from build123d import *

# Parameters (mm, degrees)
SKETCH1_W               = 36
SKETCH1_H               = 36
BOSS_EXTRUDE1_DEPTH     = 6.5
SKETCH2_R               = 14
SKETCH2_R_2             = 5.9
BOSS_EXTRUDE2_DEPTH     = 9.15
CAVITY1_START           = 5.65
CAVITY1_OUTLINE_R       = 5.4
CAVITY1_DEPTH           = 10
SKETCH5_W               = 36
SKETCH5_H               = 36
CUT_EXTRUDE1_DEPTH      = 8.55
SKETCH6_R               = 1.83
CUT_EXTRUDE2_DEPTH      = 2.1
FILLET1_R               = 1
CUT_EXTRUDE3_DEPTH      = 28.349588662
CUT_EXTRUDE3_DEPTH_BACK = 28.349588662
SKETCH7_R               = 0.665


with BuildPart() as part:
    # Sketch1 → Boss-Extrude1 (new, symmetric)
    with BuildSketch(Plane(origin=(0, 0, 0), x_dir=(1, 0, 0), z_dir=(0, 1, 0))):
        Rectangle(SKETCH1_W, SKETCH1_H)
    extrude(amount=BOSS_EXTRUDE1_DEPTH, both=True)

    # Sketch2 → Boss-Extrude2 (add)
    with BuildSketch(Plane(origin=(0, 6.5, 0), x_dir=(1, 0, 0), z_dir=(0, 1, 0))):
        with Locations(Location((0, 0, 0), (0, 0, 270))):
            Circle(SKETCH2_R)
        with Locations(Location((0, 0, 0), (0, 0, 270))):
            Circle(SKETCH2_R_2, mode=Mode.SUBTRACT)
    extrude(amount=BOSS_EXTRUDE2_DEPTH)

    # Cavity1: read off the stored shape, not the designer's step
    # Cavity1 outline → Cavity1 (cut)
    with BuildSketch(Plane(origin=(0, 0, 0), x_dir=(1, 0, 0), z_dir=(0, 1, 0)).offset(CAVITY1_START)):
        with BuildLine():
            Line((-4.533292403, -11.068981767), (-1.149066665, -7.035818585))
            ThreePointArc((-1.149066665, -7.035818585), (0.633927393, -6.640538319), (1.47721163, -8.260472267))
            Line((1.47721163, -8.260472267), (0.68813613, -12.7355418))
            ThreePointArc((0.68813613, -12.7355418), (0.138338934, -13.654010782), (-0.883764559, -13.972077877))
            ThreePointArc((-0.883764559, -13.972077877), (1.633368507, -13.904391656), (4.097662599, -13.3869026))
            ThreePointArc((4.097662599, -13.3869026), (2.691904846, -13.099521272), (2.170695102, -11.762702927))
            Line((2.170695102, -11.762702927), (2.83719432, -6.540139582))
            ThreePointArc((2.83719432, -6.540139582), (4.123439724, -5.243649297), (5.708657981, -6.150510574))
            Line((5.708657981, -6.150510574), (7.46425068, -10.341785051))
            ThreePointArc((7.46425068, -10.341785051), (7.498293668, -11.411693133), (6.810405547, -12.231859069))
            ThreePointArc((6.810405547, -12.231859069), (8.891358698, -10.814052918), (10.684679103, -9.046415448))
            ThreePointArc((10.684679103, -9.046415448), (9.346710352, -9.564664912), (8.185502249, -8.721849019))
            Line((8.185502249, -8.721849019), (5.922666155, -3.968012472))
            ThreePointArc((5.922666155, -3.968012472), (6.303789078, -2.181938673), (8.127645759, -2.087805232))
            Line((8.127645759, -2.087805232), (11.870518379, -4.664584621))
            ThreePointArc((11.870518379, -4.664584621), (12.477593142, -5.546243546), (12.342320013, -6.608111432))
            ThreePointArc((12.342320013, -6.608111432), (13.326405326, -4.290328786), (13.879385486, -1.833755311))
            ThreePointArc((13.879385486, -1.833755311), (13.03400136, -2.993095023), (11.601470268, -2.911869673))
            Line((11.601470268, -2.911869673), (7.127733334, -0.136069439))
            ThreePointArc((7.127733334, -0.136069439), (6.48272994, 1.572522062), (7.966163435, 2.63776352))
            Line((7.966163435, 2.63776352), (12.507980365, 2.493588468))
            ThreePointArc((12.507980365, 2.493588468), (13.495344957, 2.08009918), (13.955635081, 1.113664893))
            ThreePointArc((13.955635081, 1.113664893), (13.530412422, 3.59554442), (12.667485044, 5.961109181))
            ThreePointArc((12.667485044, 5.961109181), (12.583089031, 4.528761388), (11.334053449, 3.82260772))
            Line((11.334053449, 3.82260772), (6.069795541, 3.73907468))
            ThreePointArc((6.069795541, 3.73907468), (4.603449851, 4.827718154), (5.275480507, 6.525860991))
            Line((5.275480507, 6.525860991), (9.174246963, 8.860064838))
            ThreePointArc((9.174246963, 8.860064838), (10.228420101, 9.046025113), (11.138134616, 8.481860484))
            ThreePointArc((11.138134616, 8.481860484), (9.438609176, 10.339857679), (7.433747604, 11.863363627))
            ThreePointArc((7.433747604, 11.863363627), (8.137134842, 10.612768057), (7.468154743, 9.343434171))
            Line((7.468154743, 9.343434171), (3.084740551, 6.427089007))
            ThreePointArc((3.084740551, 6.427089007), (1.262606961, 6.550147844), (0.909869793, 8.342043708))
            Line((0.909869793, 8.342043708), (2.927754972, 12.413533223))
            ThreePointArc((2.927754972, 12.413533223), (3.714044133, 13.139901989), (4.78435511, 13.157125301))
            ThreePointArc((4.78435511, 13.157125301), (2.350114207, 13.801339182), (-0.160152175, 13.999083944))
            ThreePointArc((-0.160152175, 13.999083944), (1.107697836, 13.327295854), (1.231169673, 11.89778629))
            Line((1.231169673, 11.89778629), (-0.879697769, 7.074547986))
            ThreePointArc((-0.879697769, 7.074547986), (-2.479104719, 6.192951873), (-3.744618151, 7.509686489))
            Line((-3.744618151, 7.509686489), (-4.248278536, 12.02579252))
            ThreePointArc((-4.248278536, 12.02579252), (-3.979514604, 13.061952825), (-3.08842334, 13.655095799))
            ThreePointArc((-3.08842334, 13.655095799), (-5.484525418, 12.88099301), (-7.70320477, 11.690194022))
            ThreePointArc((-7.70320477, 11.690194022), (-6.273425408, 11.810501383), (-5.396703069, 10.674675328))
            Line((-5.396703069, 10.674675328), (-4.564838262, 5.475887966))
            ThreePointArc((-4.564838262, 5.475887966), (-5.433718166, 3.869537441), (-7.210216291, 4.293056871))
            Line((-7.210216291, 4.293056871), (-10.075513626, 7.819947663))
            ThreePointArc((-10.075513626, 7.819947663), (-10.409605573, 8.836925932), (-9.980649201, 9.817669863))
            ThreePointArc((-9.980649201, 9.817669863), (-11.577866975, 7.871022571), (-12.800544279, 5.669750096))
            ThreePointArc((-12.800544279, 5.669750096), (-11.66278041, 6.543956173), (-10.311160718, 6.062430373))
            Line((-10.311160718, 6.062430373), (-6.800674861, 2.138672207))
            ThreePointArc((-6.800674861, 2.138672207), (-6.663164489, 0.317572211), (-8.386621704, -0.28658797))
            Line((-8.386621704, -0.28658797), (-12.703844329, 1.131324675))
            ThreePointArc((-12.703844329, 1.131324675), (-13.534720323, 1.806237493), (-13.70408946, 2.863203114))
            ThreePointArc((-13.70408946, 2.863203114), (-13.995317572, 0.362058079), (-13.833801424, -2.150799424))
            ThreePointArc((-13.833801424, -2.150799424), (-13.349285037, -0.800248885), (-11.951897694, -0.474593391))
            Line((-11.951897694, -0.474593391), (-6.877345242, -1.877556866))
            ThreePointArc((-6.877345242, -1.877556866), (-5.777103166, -3.335219951), (-6.900333982, -4.775243156))
            Line((-6.900333982, -4.775243156), (-11.29879422, -5.916485904))
            ThreePointArc((-11.29879422, -5.916485904), (-12.362657002, -5.797918587), (-13.076578144, -5.000310394))
            ThreePointArc((-13.076578144, -5.000310394), (-11.969353727, -7.261857295), (-10.474924362, -9.288485324))
            ThreePointArc((-10.474924362, -9.288485324), (-10.797485986, -7.890380576), (-9.7979916, -6.860937106))
            Line((-9.7979916, -6.860937106), (-4.770507103, -5.2976749))
            ThreePointArc((-4.770507103, -5.2976749), (-3.056852407, -5.929103345), (-3.223238977, -7.74779238))
            Line((-3.223238977, -7.74779238), (-6.306456779, -11.085854011))
            ThreePointArc((-6.306456779, -11.085854011), (-7.265537434, -11.561276482), (-8.297345663, -11.276260681))
            ThreePointArc((-8.297345663, -11.276260681), (-6.143204645, -12.580184287), (-3.790332827, -13.477142763))
            ThreePointArc((-3.790332827, -13.477142763), (-4.817561427, -12.475372185), (-4.533292403, -11.068981767))
        make_face()
        Circle(CAVITY1_OUTLINE_R, mode=Mode.SUBTRACT)
    extrude(amount=CAVITY1_DEPTH, mode=Mode.SUBTRACT)

    # Cavity1 2 outline → Cavity1 2 (revolve, cut)
    with BuildSketch(Plane.XY):
        Polygon((14, 6.5), (14, 5.65), (14.15, 5.65), (15, 6.5), align=None)
    revolve(axis=Axis((0, 0, 0), (0, 1, 0)), mode=Mode.SUBTRACT)

    # Sketch5 → Cut-Extrude1 (cut)
    with BuildSketch(Plane.XZ.offset(6.5)):
        Rectangle(SKETCH5_W, SKETCH5_H)
    extrude(amount=-CUT_EXTRUDE1_DEPTH, mode=Mode.SUBTRACT)

    # Sketch6 → Cut-Extrude2 (cut)
    with BuildSketch(Plane(origin=(0, 6.5, 0), x_dir=(1, 0, 0), z_dir=(0, 1, 0))):
        with Locations(Location((-15.75, -15.75, 0), (0, 0, 270))):
            Circle(SKETCH6_R)
        with Locations(Location((15.75, -15.75, 0), (0, 0, 270))):
            Circle(SKETCH6_R)
        with Locations(Location((15.75, 15.75, 0), (0, 0, 270))):
            Circle(SKETCH6_R)
        with Locations(Location((-15.75, 15.75, 0), (0, 0, 270))):
            Circle(SKETCH6_R)
    extrude(amount=-CUT_EXTRUDE2_DEPTH, mode=Mode.SUBTRACT)

    # Fillet1
    fillet1_edges = [part.edges().sort_by_distance(p)[0] for p in [
        (15.75, 4.4, -17.58),
        (-15.75, 4.4, 13.92),
        (-15.75, 4.4, -17.58),
        (15.75, 4.4, 13.92),
    ]]
    fillet(fillet1_edges, radius=FILLET1_R)

    # Sketch7 → Cut-Extrude3 (cut, two sides: drawn at the far end of the back side and taken through both)
    with BuildSketch(Plane(origin=(0, 5.65, 0), x_dir=(1, 0, 0), z_dir=(0, 1, 0)).offset(-CUT_EXTRUDE3_DEPTH_BACK)):
        with Locations(Location((0, 6.4, 0), (0, 0, 270))):
            Circle(SKETCH7_R)
        with Locations(Location((2.257018876, 12.954858772, 0), (0, 0, 270))):
            Circle(SKETCH7_R)
        with Locations(Location((3.460101232, 5.38402261, 0), (0, 0, 270))):
            Circle(SKETCH7_R)
        with Locations(Location((8.90265054, 9.678084179, 0), (0, 0, 270))):
            Circle(SKETCH7_R)
        with Locations(Location((5.82164477, 2.658656083, 0), (0, 0, 270))):
            Circle(SKETCH7_R)
        with Locations(Location((12.72175356, 3.328586241, 0), (0, 0, 270))):
            Circle(SKETCH7_R)
        with Locations(Location((6.334857228, -0.910814965, 0), (0, 0, 270))):
            Circle(SKETCH7_R)
        with Locations(Location((12.501789712, -4.077714309, 0), (0, 0, 270))):
            Circle(SKETCH7_R)
        with Locations(Location((4.836797276, -4.191108697, 0), (0, 0, 270))):
            Circle(SKETCH7_R)
        with Locations(Location((8.312595965, -10.189369378, 0), (0, 0, 270))):
            Circle(SKETCH7_R)
        with Locations(Location((1.803088364, -6.140755031, 0), (0, 0, 270))):
            Circle(SKETCH7_R)
        with Locations(Location((1.484211732, -13.065971664, 0), (0, 0, 270))):
            Circle(SKETCH7_R)
        with Locations(Location((-1.803088364, -6.140755031, 0), (0, 0, 270))):
            Circle(SKETCH7_R)
        with Locations(Location((-5.815399238, -11.794220267, 0), (0, 0, 270))):
            Circle(SKETCH7_R)
        with Locations(Location((-4.836797276, -4.191108697, 0), (0, 0, 270))):
            Circle(SKETCH7_R)
        with Locations(Location((-11.26866204, -6.777887268, 0), (0, 0, 270))):
            Circle(SKETCH7_R)
        with Locations(Location((-6.334857228, -0.910814965, 0), (0, 0, 270))):
            Circle(SKETCH7_R)
        with Locations(Location((-13.144204265, 0.390377048, 0), (0, 0, 270))):
            Circle(SKETCH7_R)
        with Locations(Location((-5.82164477, 2.658656083, 0), (0, 0, 270))):
            Circle(SKETCH7_R)
        with Locations(Location((-10.846554508, 7.434699409, 0), (0, 0, 270))):
            Circle(SKETCH7_R)
        with Locations(Location((-3.460101232, 5.38402261, 0), (0, 0, 270))):
            Circle(SKETCH7_R)
        with Locations(Location((-5.105200333, 12.118557239, 0), (0, 0, 270))):
            Circle(SKETCH7_R)
    extrude(amount=CUT_EXTRUDE3_DEPTH + CUT_EXTRUDE3_DEPTH_BACK, mode=Mode.SUBTRACT)


solid = part.part
Geometry: final body of the model. Coordinates: model frame, mm. A direction names the side the tool comes from. Give positions to 0.01 mm unless a question says otherwise; leave off trailing zeros. Use CSV: the item, a comma, the result in double quotes.
1. Contact query for flat-ended pins moving along their axis: pin 1 (0.5 mm diameter, centred on x = 15.5, z = -15.5, fed in from +Y); pin 2 (4 mm diameter, centred on x = -15.75, z = 15.75, fed in from +Y); pin 3 (1.5 mm diameter, centred on x = 0, z = -6.4, fed in from +Y). Output: stop coordinate, or through.
Answers below:
pin 1,"y = 4.4"
pin 2,"y = 6.5"
pin 3,"y = 5.65"
2. Material intervals for line 1 along X through (y, z) = (6.2, -15.75); line 2 along X through (y, z) = (3.75, 13); line 3 along X through (y, z) = (14.5, 7), sorted ascending. Write a range as from..to.
Answers below:
line 1,"-18..-17.58, -13.92..13.92, 17.58..18"
line 2,"-18..0.82, 2.15..18"
line 3,"-10.11..-2.85, -1.12..1.12, 2.78..6.06, 7.37..12.12"
3. Mould query, pull axis Z, two halves, no side actions, for faces 1 (the face through (0, 4, 18)), 2 (the face through (1.1, 10.58, -13.34)), 3 (the face through (-2, 15.65, 10)). Classes: +Z half, -Z half, draft (parallel to the pull), parting line (faces both ways), or undercut.
Answers below:
face 1,"+Z half"
face 2,"undercut"
face 3,"draft"
4. Section query A-A (y = 14.25). Give the number of separate pieces and of enclosed holes in the cut face, plus the area to 3 significant figures.
Answers below:
separate pieces,"11"
enclosed holes,"0"
area,"350 mm2"
5. Access query for faces 4 (the face through (12.702, 3.825, 4.712)), 5 (the face through (1.905, 10.58, -10.349)). Directions: +Z, -Z, +X, -X, +Y, -Y. A direction counts if a zero-diameter tool reaches every point of the face in a straight line with its end or side. Return the directions, or none.
Answers below:
face 4,"+Y, -Y"
face 5,"+Y"
